Can you work these out from the drawing? Everything is in mm from the part's minimum corner. Give positions to 0.01 mm unless a question says otherwise; leave off trailing zeros. Write each loop counter-clockwise with the first axis right and the second up, starting at its lowest first coordinate (ties: lowest second). Pieces come first, ordered by that corner, then holes. Notation, with made-up numbers: (-24, 41.5) -> (17, 41.5) arc R7 ccw to (17, 53.5) -> close; hole circle Ø2 at (-3.75, 69.5). An arc over 180 degrees is marked (long way). Write item = value, one per line. Start each with the question number.
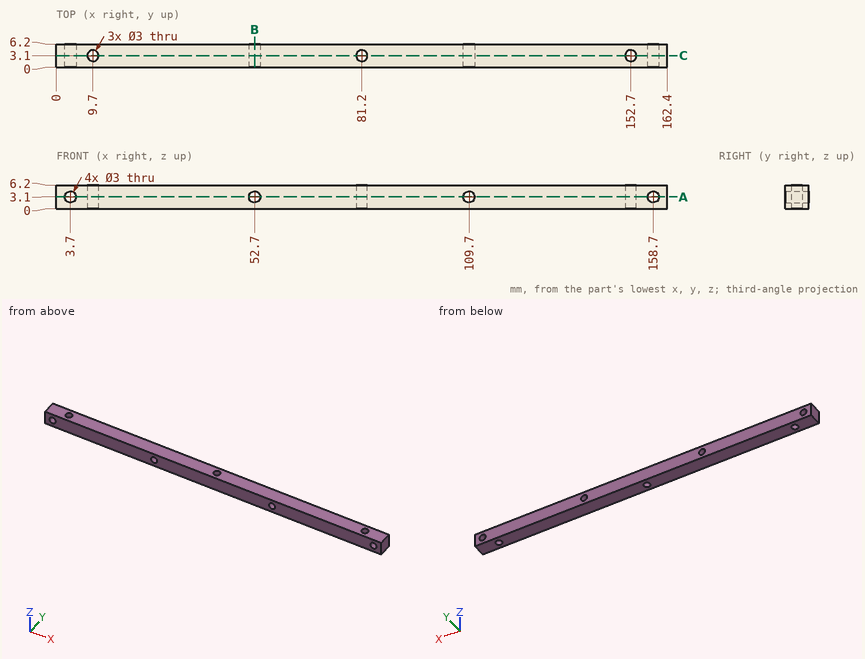
(1) If I drill on line 1 along X through (y, z) = (5.25, 2); line 2 along Z through (x, y) = (109.7, 1.5), over which ranges is the centre line in solid material (lowest first)? Write a range as from..to.
(2) Imagine slicing it at C-C (y = 3.1). Please give me the cut outline in (x, z).
(3) I'm going to push flat-ended pins straight in: pin 1 (2.5 mm diameter, centred on x = 9.7, y = 3.1, fed in from -Z); pin 2 (1 mm diameter, centred on x = 20.5, z = 2.5, fed in from -Y). Where does each tip first touch, or does it pass through?
(4) Imagine slicing it at B-B (x = 52.7). Please give me the cut outline in (y, z), then the cut area to 3 significant figures.
(5) Imagine slicing it at A-A (z = 3.1). Please give me the cut outline in (x, y).
Answers below:
q1.line_1 = 0..2.68, 4.72..51.68, 53.72..108.68, 110.72..157.68, 159.72..162.4
q1.line_2 = 0..1.6, 4.6..6.2
q2.outline = (0, 0) -> (8.2, 0) -> (8.2, 6.2) -> (0, 6.2) -> close; (11.2, 0) -> (79.7, 0) -> (79.7, 6.2) -> (11.2, 6.2) -> close; (82.7, 0) -> (151.2, 0) -> (151.2, 6.2) -> (82.7, 6.2) -> close; (154.2, 0) -> (162.4, 0) -> (162.4, 6.2) -> (154.2, 6.2) -> close; hole circle Ø3 at (3.7, 3.1); hole circle Ø3 at (52.7, 3.1); hole circle Ø3 at (109.7, 3.1); hole circle Ø3 at (158.7, 3.1)
q3.pin_1 = through
q3.pin_2 = 0
q4.outline = (0, 0) -> (6.2, 0) -> (6.2, 1.6) -> (0, 1.6) -> close; (0, 4.6) -> (6.2, 4.6) -> (6.2, 6.2) -> (0, 6.2) -> close
q4.area = 19.8 mm^2
q5.outline = (0, 0) -> (2.2, 0) -> (2.2, 6.2) -> (0, 6.2) -> close; (5.2, 0) -> (51.2, 0) -> (51.2, 6.2) -> (5.2, 6.2) -> close; (54.2, 0) -> (108.2, 0) -> (108.2, 6.2) -> (54.2, 6.2) -> close; (111.2, 0) -> (157.2, 0) -> (157.2, 6.2) -> (111.2, 6.2) -> close; (160.2, 0) -> (162.4, 0) -> (162.4, 6.2) -> (160.2, 6.2) -> close; hole circle Ø3 at (9.7, 3.1); hole circle Ø3 at (81.2, 3.1); hole circle Ø3 at (152.7, 3.1)
